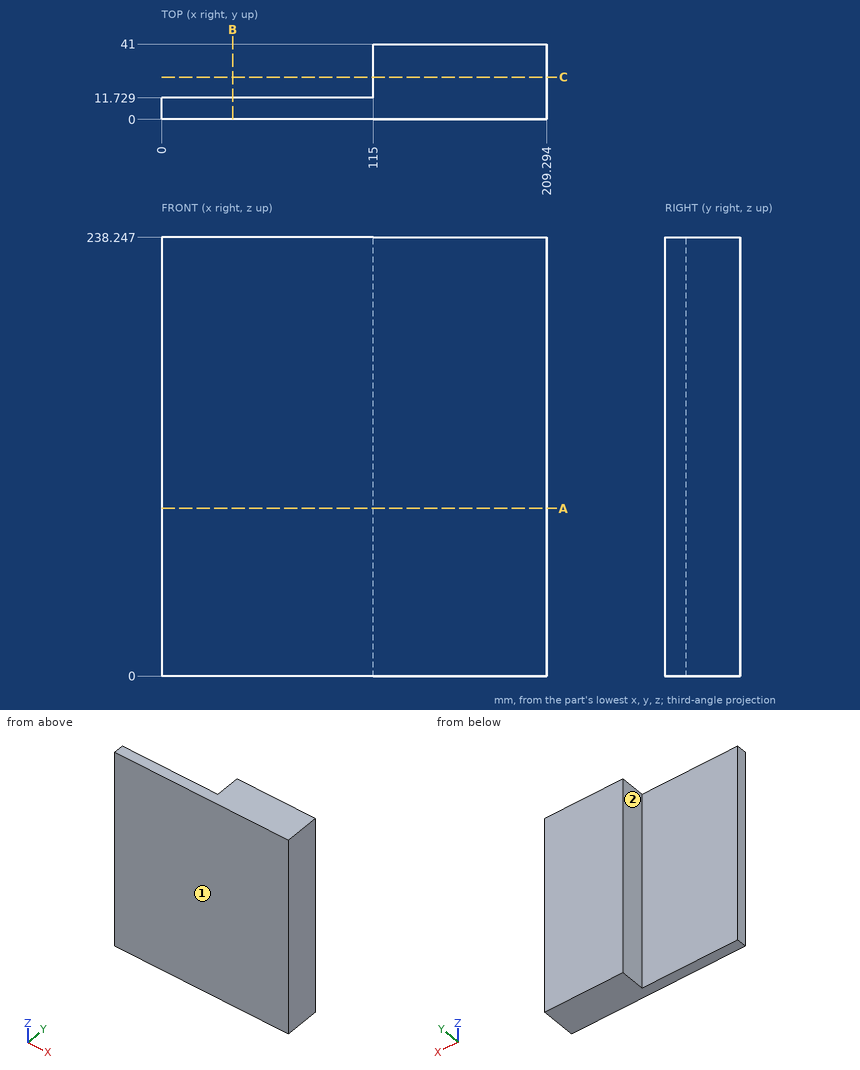
Design review of the part shown in the three views and the two pictorial views. Dimensions are in mm from the part's minimum x, y and z. A direction names the side the tool comes from. Coordinates: 2 decimals unless noted, no trailing zeros. Order: outer loops, then holes, each group sorted by start corner. A loop starts at its lowest first (then second) coordinate and runs counter-clockwise, first axis right, second up.
1) For the marked faces 1 and 2, list the 3-axis set-ups (+Z, -Z, +X, -X, +Y, -Y) from which the entire face can be reached by the end or side of a thin tool; tool diameter is ignored.
2) Take a section at C-C, the plane y = 23. Give the boundary of the cut face in (x, z) (1 decimal).
3) Clearance check with flat-ended pins moving along their axes: pin 1 (23.5 mm diameter, centred on y = 20.5, z = 59.5, fed in from -X); pin 2 (10 mm diameter, centred on y = 26, z = 174.5, fed in from -X); pin 3 (6 mm diameter, centred on x = 27, z = 125, fed in from +Y). State where each tip first meets the part, or that it passes through.
4) Take a section at A-A, the plane z = 91. Give the boundary of the cut face in (x, y) (1 decimal).
5) Wall thickness on line 1 along X through (y, z) = (24.5, 203.5) (1 decimal); line 2 along Y through (x, z) = (29, 194): over which ranges is each line inside the solid? List them lowest first.
6) Take a section at B-B, the plane x = 38.5. Give the boundary of the cut face in (y, z).
Returned:
1. face 1: +Z, -Z, +X, -X, -Y
1. face 2: +Z, -Z, -X, +Y
2. outline: (115, 0) - (209.3, 0) - (209.3, 238.2) - (115, 238.2) - close
3. pin 1: stops at x = 0
3. pin 2: stops at x = 115
3. pin 3: stops at y = 11.73
4. outline: (0, 0) - (209.3, 0) - (209.3, 41) - (115, 41) - (115, 11.7) - (0, 11.7) - close
5. line 1: x = 115 to 209.3
5. line 2: y = 0 to 11.73
6. outline: (0, 0) - (11.73, 0) - (11.73, 238.25) - (0, 238.25) - close
